Geometry check sheet. Reference: the model listing, model coordinates, mm. A direction names the side the tool comes from. Round coordinates to 2 decimals unless told otherwise and drop trailing zeros. Order: outer loops, then holes, each group sorted by start corner. A loop starts at its lowest first (then second) coordinate and runs counter-clockwise, first axis right, second up.
(1) Cross-section at C-C on x = 13.5. Enter the section's corners in (y, z).
(2) Set-up check for faces 4 (the face through (24.3, -88.7, -16)), 5 (the face through (16, -37, -3)), 6 (the face through (30, -1, -11)): record each of +Z, -Z, +X, -X, +Y, -Y from which the full face is reachable in a straight line by a thin tool's end or side.
(3) Cross-section at B-B on z = -11.25. Enter the section's corners in (x, y), and give its area (3 significant figures).
(4) Cross-section at D-D on y = 38. Enter the section's corners in (x, z), and give its area (3 significant figures).
(5) Thickness scan on L1, parallel to X at y = -90, z = -19.55; L2, parallel to X at y = -90, z = -4.5; L3, parallel to Y at x = -12, z = -11. Record the ranges inside material, lowest first.
(6) Gauge pin test, flat ends, axial feed: P1, Ø8, axis at x = 16, y = -3, coming from the +Z side; P2, Ø5, axis at x = -12, y = -90, coming from the -Z side. Record the tip position at first contact, or that the pin passes through.
(7) Cross-section at A-A on y = -19. Enter the section's corners in (x, z), and give its area (3 significant figures).
(8) Draft check along X on faces 1 (the face through (-20, -1, -11)), 2 (the face through (5, -100, -11)), 3 (the face through (-0.1, -75, -3.4)). Enter one of: pulls with the +X half, pulls with the -X half, needs draft (parallel to the pull), parting line crosses it, or undercut.
from build123d import *

# Parameters (mm, degrees)
SKETCH006_R     = 3.009992
PAD002_DEPTH    = 100
SKETCH011_R     = 5
PAD007_DEPTH    = 50
SKETCH010_R     = 5
PAD006_DEPTH    = 50
SKETCH008_R     = 13
PAD004_DEPTH    = 15
SKETCH009_R     = 9
PAD005_DEPTH    = 15
SKETCH013_R     = 6
PAD008_DEPTH    = 26
BOX001_W        = 50
BOX001_H        = 200
BOX001_DEPTH    = 20
SKETCH015_R     = 1.5
POCKET001_DEPTH = 434.247304
SKETCH016_R     = 1.5
POCKET002_DEPTH = 434.247304
SKETCH017_R     = 3
POCKET003_DEPTH = 5
SKETCH018_R     = 3
POCKET004_DEPTH = 5


with BuildPart() as pad002:
    # Sketch006 → Pad002 (new body, symmetric)
    with BuildSketch(Plane.XZ):
        Circle(SKETCH006_R)
    extrude(amount=PAD002_DEPTH, both=True)


with BuildPart() as pad007:
    # Sketch011 → Pad007 (new body)
    with BuildSketch(Plane.XZ.offset(-75)):
        Circle(SKETCH011_R)
    extrude(amount=PAD007_DEPTH)


with BuildPart() as scassi_perno:
    # Sketch010 → Pad006 (new body)
    with BuildSketch(Plane.XZ.offset(25)):
        Circle(SKETCH010_R)
    extrude(amount=PAD006_DEPTH)

    # Fusion002: union Pad007
    add(pad007.part)


with BuildPart() as scasso_ruota_dentata:
    # Sketch008 → Pad004 (new body)
    with BuildSketch(Plane.XZ.offset(-3)):
        Circle(SKETCH008_R)
    extrude(amount=PAD004_DEPTH)


with BuildPart() as obj1:
    # Sketch009 → Pad005 (new body)
    with BuildSketch(Plane.XZ.offset(-3)):
        with Locations((15.997087, 9e-06)):
            Circle(SKETCH009_R)
    extrude(amount=PAD005_DEPTH)

    # Fusion001: union scasso_ruota_dentata
    add(scasso_ruota_dentata.part)


with BuildPart() as fusion:
    # Sketch013 → Pad008 (new body)
    with BuildSketch(Plane.XZ.offset(11)):
        with Locations((16.059561, 9e-06)):
            Circle(SKETCH013_R)
    extrude(amount=PAD008_DEPTH)

    # Fusion005: union scassi_perno, obj1
    add(scassi_perno.part)
    add(obj1.part)

    # Fusion: union Pad002
    add(pad002.part)


with BuildPart() as obj2:
    # Box001 → Box001 (new body)
    with BuildSketch(Plane(origin=(-20, -100, -21), x_dir=(1, 0, 0), z_dir=(0, 0, 1))):
        with Locations((25, 100)):
            Rectangle(BOX001_W, BOX001_H)
    extrude(amount=BOX001_DEPTH)

    # Cut001: cut Fusion
    add(fusion.part, mode=Mode.SUBTRACT)

    # Sketch015 → Pocket001 (cut, through all)
    with BuildSketch(Plane(origin=(0, 0, -21), x_dir=(1, 0, 0), z_dir=(0, 0, -1))):
        with Locations((23, 90)):
            Circle(SKETCH015_R)
    pocket001 = extrude(amount=-POCKET001_DEPTH, mode=Mode.SUBTRACT)

    # Mirrored: Pocket001 across Sketch015 H_Axis
    add(pocket001.mirror(Plane(origin=(0, 0, -21), x_dir=(0, 0, -1), z_dir=(0, -1, 0))), mode=Mode.SUBTRACT)

    # Sketch016 → Pocket002 (cut, through all)
    with BuildSketch(Plane(origin=(0, 0, -21), x_dir=(1, 0, 0), z_dir=(0, 0, -1))):
        with Locations((-12, 90)):
            Circle(SKETCH016_R)
    pocket002 = extrude(amount=-POCKET002_DEPTH, mode=Mode.SUBTRACT)

    # Mirrored001: Pocket002 across Sketch016 H_Axis
    add(pocket002.mirror(Plane(origin=(0, 0, -21), x_dir=(0, 0, -1), z_dir=(0, -1, 0))), mode=Mode.SUBTRACT)

    # Sketch017 → Pocket003 (cut)
    with BuildSketch(Plane(origin=(0, 0, -21), x_dir=(1, 0, 0), z_dir=(0, 0, -1))):
        with Locations((23, 90)):
            Circle(SKETCH017_R)
    pocket003 = extrude(amount=-POCKET003_DEPTH, mode=Mode.SUBTRACT)

    # Mirrored002: Pocket003 across Sketch017 H_Axis
    add(pocket003.mirror(Plane(origin=(0, 0, -21), x_dir=(0, 0, -1), z_dir=(0, -1, 0))), mode=Mode.SUBTRACT)

    # Sketch018 → Pocket004 (cut)
    with BuildSketch(Plane(origin=(0, 0, -21), x_dir=(1, 0, 0), z_dir=(0, 0, -1))):
        with Locations((-12, 90)):
            Circle(SKETCH018_R)
    pocket004 = extrude(amount=-POCKET004_DEPTH, mode=Mode.SUBTRACT)

    # Mirrored003: Pocket004 across Sketch018 H_Axis
    add(pocket004.mirror(Plane(origin=(0, 0, -21), x_dir=(0, 0, -1), z_dir=(0, -1, 0))), mode=Mode.SUBTRACT)


solid = obj2.part
Found:
1. outline: (-100, -21) - (100, -21) - (100, -1) - (3, -1) - (3, -8.65) - (-12, -8.65) - (-12, -5.43) - (-37, -5.43) - (-37, -1) - (-100, -1) - close
2. face 4: -Z
2. face 5: +Z
2. face 6: +Z, -Z, +X, +Y, -Y
3. outline: (-20, -100) - (30, -100) - (30, 100) - (-20, 100) - close; hole circle Ø3 at (-12, -90); hole circle Ø3 at (-12, 90); hole (-6.51, -12) - (6.51, -12) - (6.51, 3) - (-6.51, 3) - close; hole circle Ø3 at (23, -90); hole circle Ø3 at (23, 90)
3. area: 9,780 mm2
4. outline: (-20, -21) - (30, -21) - (30, -1) - (4.9, -1) arc R5 cw to (-4.9, -1) - (-20, -1) - close
4. area: 971 mm2
5. L1: x = -20 to -15, -9 to 20, 26 to 30
5. L2: x = -20 to -13.5, -10.5 to 21.5, 24.5 to 30
5. L3: y = -100 to -91.5, -88.5 to 88.5, 91.5 to 100
6. P1: stops at z = -8.06
6. P2: stops at z = -16
7. outline: (-20, -21) - (30, -21) - (30, -1) - (21.98, -1) arc R6 cw to (10.14, -1) - (2.84, -1) arc R3.01 cw to (-2.84, -1) - (-20, -1) - close
7. area: 947 mm2
8. face 1: pulls with the -X half
8. face 2: needs draft
8. face 3: undercut
